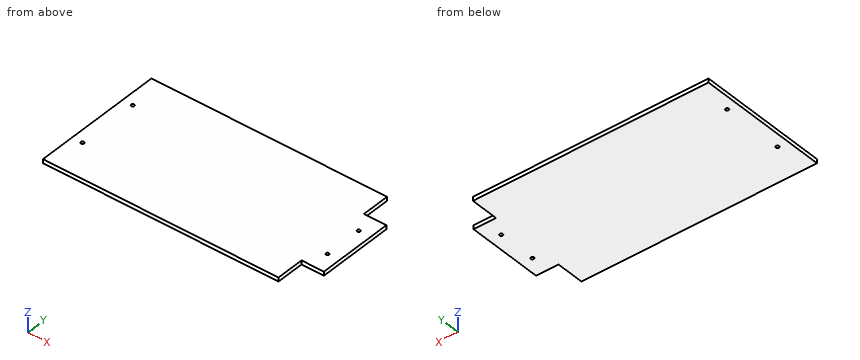
```python
from build123d import *

# Parameters (mm, degrees)
BOSS_EXTRUDE1_DEPTH = 5
SKETCH2_R           = 2
CUT_EXTRUDE1_DEPTH  = 10


with BuildPart() as part:
    # Sketch1 → Boss-Extrude1 (new body)
    with BuildSketch(Plane.XY):
        Polygon((-164.220930233, -82.5), (-164.220930233, 82.5), (130.179069767, 82.5), (130.179069767, 47.5), (158.179069767, 47.5), (158.179069767, -47.5), (130.179069767, -47.5), (130.179069767, -82.5), align=None)
    extrude(amount=BOSS_EXTRUDE1_DEPTH)

    # Sketch2 → Cut-Extrude1 (cut)
    with BuildSketch(Plane.XY.offset(5)):
        with Locations((-151.220930233, 38.25)):
            Circle(SKETCH2_R)
        with Locations((-151.220930233, -38.25)):
            Circle(SKETCH2_R)
        with Locations((143.179069767, 23.75)):
            Circle(SKETCH2_R)
        with Locations((143.179069767, -23.75)):
            Circle(SKETCH2_R)
    extrude(amount=-CUT_EXTRUDE1_DEPTH, mode=Mode.SUBTRACT)


solid = part.part
```
Source: CAD feature listing. Evaluate the final solid. Frame: model axes, mm. Give positions to 0.01 mm unless a question says otherwise; leave off trailing zeros. Loops run counter-clockwise (first coordinate to the right, second up) from the corner with the lowest first, then second, coordinate; pieces in that order, holes last. Notation, with made-up numbers: M 39.5,21.5 L 75.5,21.5 A20 ccw 75.5,51.5 Z; hole C 29.5,87.25 d7. An arc over 180 degrees is marked long. Put each result on its own line as item: value.
Q1. Line query: probe 1 along X at (y, z) = (38.5, 1.4); probe 2 along X at (y, z) = (-58.5, 4.2). Output: solid intervals per line, ascending. Write a range as [from, to].
Response values:
probe 1: x = [-164.22, -153.21], [-149.24, 158.18]
probe 2: x = [-164.22, 130.18]
Q2. Section A-A (z = 2.95). Return the cut outline in (x, y), and give its area (3 significant figures).
Response values:
outline: M -164.22,-82.5 L 130.18,-82.5 L 130.18,-47.5 L 158.18,-47.5 L 158.18,47.5 L 130.18,47.5 L 130.18,82.5 L -164.22,82.5 Z; hole C -151.22,-38.25 d4; hole C -151.22,38.25 d4; hole C 143.18,-23.75 d4; hole C 143.18,23.75 d4
area: 51,200 mm²
Q3. Pin query (flat end, axial travel): P1, Ø2.5, axis at y = -56.5, z = 3.5, coming from the +X side; P2, Ø2.5, axis at x = -151.22, y = -38.25, coming from the -Z side. Return the tip coordinate at first contact, or that it passes through.
Response values:
P1: stops at x = 130.18
P2: passes through
Q4. Section B-B (y = -53). Return the cut outline in (x, z).
Response values:
outline: M -164.22,0 L 130.18,0 L 130.18,5 L -164.22,5 Z
